Design review of the part shown in the three views and the two pictorial views. Dimensions are in mm from the part's minimum x, y and z. A direction names the side the tool comes from. Coordinates: 2 decimals unless noted, no trailing zeros. Loops run counter-clockwise (first coordinate to the right, second up) from the corner with the lowest first, then second, coordinate; pieces in that order, holes last. Notation, with made-up numbers: (13.25, 84.25) - (64.25, 84.25) arc R29 cw to (64.25, 117.25) - close; hole circle Ø4 at (-21.75, 70.5). An arc over 180 degrees is marked (long way). One line per item, written item: value. Start each with the question number.
1. Take a section at B-B, the plane y = 16. State the section outline as (x, z) points (1 decimal).
2. The part is to be moulded in two halves that separate along Z. For the marked faces 3 and 4, say which applies: released by +Z, released by -Z, zero draft, split by the parting line, or undercut.
3. Take a section at A-A, the plane y = 3.85. State the section outline as (x, z) points.
4. To check wall thickness, follow line 1 (X direction, y = 33, z = 2.5) (1 decimal); line 2 (Y direction, x = 80, z = 2.5); line 3 (Z direction, x = 59.5, y = 33). State the ranges of each line that lie inside material, in increasing order. Write a range as from..to.
5. Take a section at D-D, the plane y = 29. State the section outline as (x, z) points (1 decimal).
6. For the marked faces 1 and 2, list the 3-axis set-ups (+Z, -Z, +X, -X, +Y, -Y) from which the entire face can be reached by the end or side of a thin tool; tool diameter is ignored.
7. Insertion check: pin 1 (5 mm diameter, centred on x = 93, y = 32.5, fed in from +Z); pin 2 (2 mm diameter, centred on x = 21, z = 3, fed in from +Y); pin 3 (3.5 mm diameter, centred on x = 11, z = 3, fed in from -Y); pin 4 (6 mm diameter, centred on x = 46.5, y = 7, fed in from -Z). Each pin has a flat end and moves straight along its axis. Give the tip position at first contact, or say it passes through.
8. Take a section at C-C, the plane x = 81.5. State the section outline as (y, z) points.
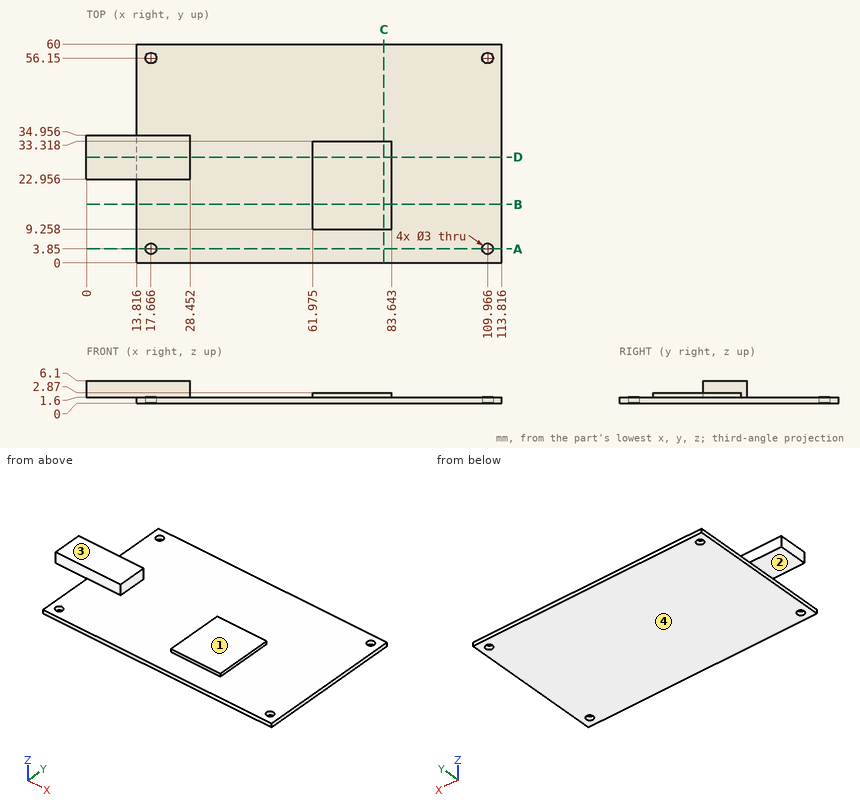
Solutions:
1. outline: (13.8, 0) - (113.8, 0) - (113.8, 1.6) - (83.6, 1.6) - (83.6, 2.9) - (62, 2.9) - (62, 1.6) - (13.8, 1.6) - close
2. face 3: released by +Z
2. face 4: released by -Z
3. outline: (13.82, 0) - (16.17, 0) - (16.17, 1.6) - (13.82, 1.6) - close; (19.17, 0) - (108.47, 0) - (108.47, 1.6) - (19.17, 1.6) - close; (111.47, 0) - (113.82, 0) - (113.82, 1.6) - (111.47, 1.6) - close
4. line 1: 0..28.5, 62..83.6
4. line 2: 9.26..33.32
4. line 3: 0..1.6
5. outline: (0, 1.6) - (13.8, 1.6) - (13.8, 0) - (113.8, 0) - (113.8, 1.6) - (83.6, 1.6) - (83.6, 2.9) - (62, 2.9) - (62, 1.6) - (28.5, 1.6) - (28.5, 6.1) - (0, 6.1) - close
6. face 1: +Z, +X, +Y, -Y
6. face 2: -Z, -X, +Y, -Y
7. pin 1: z = 1.6
7. pin 2: y = 34.96
7. pin 3: y = 22.96
7. pin 4: z = 0
8. outline: (0, 0) - (60, 0) - (60, 1.6) - (33.32, 1.6) - (33.32, 2.87) - (9.26, 2.87) - (9.26, 1.6) - (0, 1.6) - close
